Check sheet for the modelled part. Datum: model origin and axes. Units: mm. Face numbers are marked on the shaded views. A direction names the side the tool comes from. Round coordinates to 2 decimals unless told otherwise and drop trailing zeros. Order: outer loops, then holes, each group sorted by start corner. A loop starts at its lowest first (then second) coordinate and runs counter-clockwise, first axis right, second up.
Q1. Scan lines: probe 1 along X at (y, z) = (-57, 22.5); probe 2 along Z at (x, y) = (-79, 9); probe 3 along X at (y, z) = (1, 39). Record each from-to range of solid material in increasing order.
Q2. Cross-section at B-B on x = -5. Record the cut outline in (y, z), then the cut area to 3 significant figures.
Q3. Set-up check for the marked faces 1 and 2: record each of +Z, -Z, +X, -X, +Y, -Y from which the full face is reachable in a straight line by a thin tool's end or side.
Q4. Depth check by flat-ended pin: P1, Ø8, axis at x = 14.5, y = -28.5, coming from the -Z side; P2, Ø3, axis at y = -25.5, z = 43, coming from the +X side; P3, Ø10, axis at y = -21, z = -40, coming from the -X side. Enter the tip coordinate at first touch or a pass-through.
Q5. Cross-section at A-A on x = -110. Record the cut outline in (y, z), then the cut area to 3 significant figures.
from build123d import *

# Parameters (mm, degrees)
F2_DEPTH = 25.4
F3_R     = 18.5543497172
F4_DEPTH = 101.6
F5_R     = 5.08
F6_R     = 5.08
F7_R     = 5.08


with BuildPart() as f1:
    # F0 (on Front) → F1 (revolve)
    with BuildSketch(Plane.XZ):
        Polygon((0, 65.1774853468), (0, 0), (57.9038485885, 0), align=None)
    revolve(axis=Axis((28.9519242942, 0, 0), (1, 0, 0)))

    # F2 (add): a face of the model
    f2_faces = [f1.faces().sort_by_distance(p)[0] for p in [
        (0, 0, 0),
    ]]
    extrude(f2_faces, amount=F2_DEPTH)

    # F3 (on face) → F4 (join)
    with BuildSketch(Plane(origin=(-25.4, 0, 0), x_dir=(0, -1, 0), z_dir=(-1, 0, 0))):
        Circle(F3_R)
    extrude(amount=F4_DEPTH)

    # F5
    f5_edges = [f1.edges().sort_by_distance(p)[0] for p in [
        (0, 0, -65.177485),
    ]]
    fillet(f5_edges, radius=F5_R)

    # F6
    f6_edges = [f1.edges().sort_by_distance(p)[0] for p in [
        (-25.4, 0, -65.177485),
    ]]
    fillet(f6_edges, radius=F6_R)

    # F7
    f7_edges = [f1.edges().sort_by_distance(p)[0] for p in [
        (-127, 18.55435, 0),
    ]]
    fillet(f7_edges, radius=F7_R)


solid = f1.part
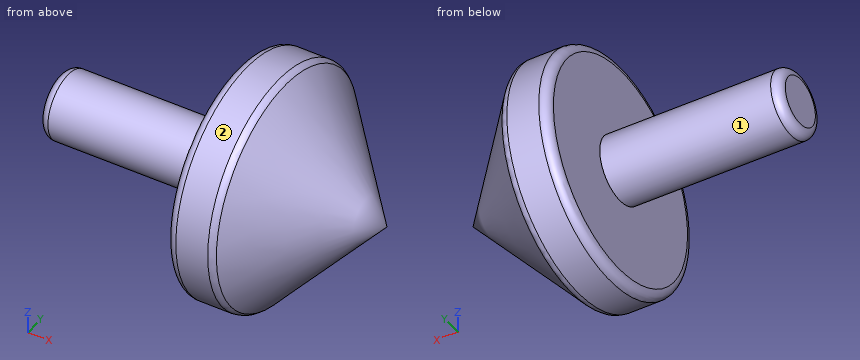
Results found:
1. probe 1: x = -25.26 to 3.46
1. probe 2: z = -16.23 to 16.23
1. probe 3: x = -25.4 to 23.24
2. outline: circle Ø130.35 at (0, 0)
2. area: 13,300 mm2
3. face 1: -X
3. face 2: +X, -X
4. P1: stops at z = -45.65
4. P2: stops at x = 14.82
4. P3: stops at x = -25.4
5. outline: circle Ø37.11 at (0, 0)
5. area: 1,080 mm2
